Check sheet for the modelled part. Datum: model origin and axes. Units: mm. Face numbers are marked on the shaded views. Round coordinates to 2 decimals unless told otherwise and drop trailing zeros. Write each loop counter-clockwise with the first axis right and the second up, starting at its lowest first coordinate (ties: lowest second). Pieces come first, ordered by that corner, then holes. Notation, with made-up numbers: (-10.75, -24.5) -> (43.25, -24.5) arc R34 ccw to (43.25, 6.5) -> close; hole circle Ø2 at (16, 59.25). An arc over 180 degrees is marked (long way). Use one line per item in the form item = value. Start each with the question number.
Autodesk Inventor part; units mm, degrees
ref_plane "Work Plane2" through (6, 0, 86) normal (0, 0, 1) x (0, 1, 0)
ref_plane "YZ Plane" through (0, 0, 0) normal (1, 0, 0) x (0, 1, 0)
ref_plane "XZ Plane" through (0, 0, 0) normal (0, 1, 0) x (-1, 0, 0)
sketch "Sketch1" plane through (0, 0, 0) normal (0, 1, 0) x (-1, 0, 0)
  circle A0 centre (0, 0) radius 6
  line L0 (0, 0) -> (0, 90) construction
  circle A1 centre (0, 90) radius 6
  line L1 (12.9035, -6) -> (-17.4473, -6) construction
  line L2 (12.9035, 96) -> (-17.4473, 96) construction
  line L3 (6, 90) -> (6, 0)
  line L4 (-6, 90) -> (-6, 0)
  line L5 (12.9035, 10) -> (-17.4473, 10) construction
  line L6 (12.7918, 80) -> (-17.559, 80) construction
  circle A2 centre (0, 77.5) radius 2.5
  circle A3 centre (0, 12.5) radius 2.5
  line L7 (2.5, 77.5) -> (2.5, 12.5)
  line L8 (-2.5, 12.5) -> (-2.5, 77.5)
  dimension "d0" = 12
  dimension "d1" = 12
  dimension "d2" = 102
  dimension "d3" = 70
  dimension "d4" = 16
  dimension "d5" = 5
  dimension "d6" = 5
extrude "Extrusion1" add sketch "Sketch1" along normal blind 1.5
ref_plane "Work Plane2" through (6, 0, 86) normal (0, 0, 1) x (0, 1, 0)
ref_plane "Work Plane1" through (6, 0, 90) normal (0, 0, 1) x (0, 1, 0)
sketch "Sketch2" plane through (6, 0, 86) normal (0, 0, 1) x (0, 1, 0)
  line L0 (1.5, 0) -> (1.5, 12)
  line L1 (-1.5, -2.125) -> (1.5, -2.125) construction
  line L2 (1.5, -2.125) -> (1.5, 14.125) construction
  line L3 (1.5, 14.125) -> (-1.5, 14.125) construction
  line L4 (-1.5, 14.125) -> (-1.5, -2.125) construction
  line L5 (0, 12) -> (1.5, 12)
  line L6 (0, 12) -> (0, 0)
  line L7 (0, 0) -> (1.5, 0)
  line L8 (1.5, 12) -> (1.5, 0)
  line L9 (0, 12) -> (1.5, 12)
  arc A0 (1.5, 12) -> (-0.9425, 14.125) centre (-0.6456, 12) ccw
  arc A1 (0, 12) -> (-1.5, 13.5675) centre (-1.569, 12) ccw
  line L10 (-1.5, 13.5675) -> (-0.9425, 14.125)
  line L11 (0, 0) -> (0, 12)
  line L12 (0, 6) -> (-3.8255, 6) construction
  arc A2 (-0.9425, -2.125) -> (1.5, 0) centre (-0.6456, 0) ccw
  arc A3 (-1.5, -1.5675) -> (0, 0) centre (-1.569, 0) ccw
  line L13 (-1.5, -1.5675) -> (-0.9425, -2.125)
  dimension "d11" = 3
  dimension "d12" = 16.25
  dimension "d13" = 2.125
  dimension "d15" = 1.5
  dimension "d16" = 45
extrude "Extrusion2" add sketch "Sketch2" against normal blind 82 contours A2 L13 A3 L7 | L5 A1 L10 A0
sketch "Sketch3" plane through (0, 1.5, 0) normal (0, 1, 0) x (1, 0, 0)
  arc A0 (-6, -90) -> (6, -90) centre (0, -90) ccw
  circle A1 centre (0, -90) radius 9
  point P0 (0, 0)
  dimension "d19" = 18
extrude "Extrusion3" add sketch "Sketch3" along normal blind 6.75
sketch "Sketch4" plane through (0, 8.25, 90) normal (0, 1, 0) x (1, 0, 0)
  circle A0 centre (0, 0) radius 4
  point P0 (0, 90)
  dimension "d22" = 8
extrude "Extrusion4" add sketch "Sketch4" along normal blind 1
equation "\"d1\" = d0"
equation "\"d6\" = d5"
properties part number "High Voltage Limit Switch Arm"
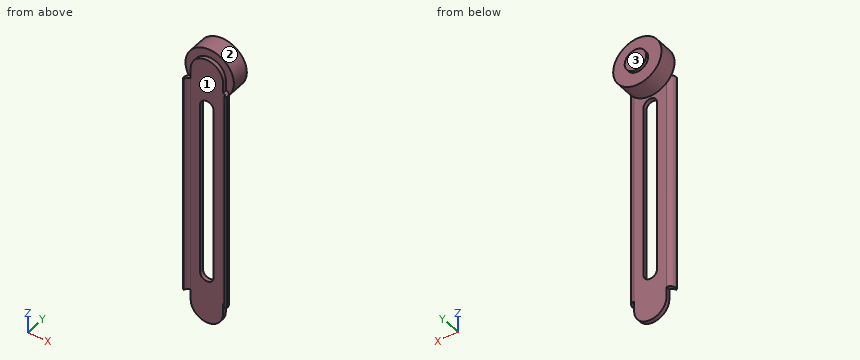
1. Depth check by flat-ended pin: pin 1 (1.6 mm diameter, centred on y = 1, z = 60, fed in from +X); pin 2 (6 mm diameter, centred on x = -2, z = 54, fed in from -Y); pin 3 (0.6 mm diameter, centred on x = 7, y = -0.5, fed in from -Z); pin 4 (9 mm diameter, centred on x = 3.5, z = 94.5, fed in from +Y). Enter the tip coordinate at first touch or a pass-through.
2. Sectioned sample at D-D (y = 3.25). Enter the section's corners in (x, z), and give its area (3 significant figures).
3. Sectioned sample at B-B (z = 79). Enter the section's corners in (x, y) (1 decimal).
4. Sectioned sample at C-C (x = 5). Enter the section's corners in (y, z), and give its area (3 significant figures).
5. Mould release check, pull along X, two halves, no side actions. Record for the marked faces 1, 2 and 3: +X half, -X half, draft (parallel to the pull), parting line (faces both ways), or undercut.
6. Scan lines: probe 1 along Y at (x, z) = (-0.5, 10); probe 2 along Y at (x, z) = (4, 94); probe 3 along Z at (x, y) = (-0.5, 6.75). Record each from-to range of solid material in increasing order.
7. Sectioned sample at A-A (x = 0). Enter the section's corners in (y, z).
Returned:
q1.pin_1 = 7.97
q1.pin_2 = 0
q1.pin_3 = 4
q1.pin_4 = 9.25
q2.outline = circle Ø18 at (0, 90)
q2.area = 254 mm^2
q3.outline = (-8.1, -0.9) -> (-7.6, -1.5) arc R1.6 cw to (-6, 0) -> (-2, 0) -> (-2, 1.5) -> (-6, 1.5) arc R2.1 ccw to start; (2, 0) -> (6, 0) arc R1.6 cw to (7.6, -1.5) -> (8.1, -0.9) arc R2.1 ccw to (6, 1.5) -> (2, 1.5) -> close
q4.outline = (0, -3.32) -> (1.5, -3.32) -> (1.5, 82.52) -> (8.25, 82.52) -> (8.25, 97.48) -> (1.5, 97.48) -> (1.5, 93.32) -> (0, 93.32) -> close
q4.area = 246 mm^2
q5.face_1 = undercut
q5.face_2 = parting line
q5.face_3 = draft
q6.probe_1 = 0 to 1.5
q6.probe_2 = 0 to 8.25
q6.probe_3 = 81.01 to 98.99
q7.outline = (0, -6) -> (1.5, -6) -> (1.5, 10) -> (0, 10) -> close; (0, 80) -> (1.5, 80) -> (1.5, 81) -> (8.25, 81) -> (8.25, 86) -> (9.25, 86) -> (9.25, 94) -> (8.25, 94) -> (8.25, 99) -> (1.5, 99) -> (1.5, 96) -> (0, 96) -> close
